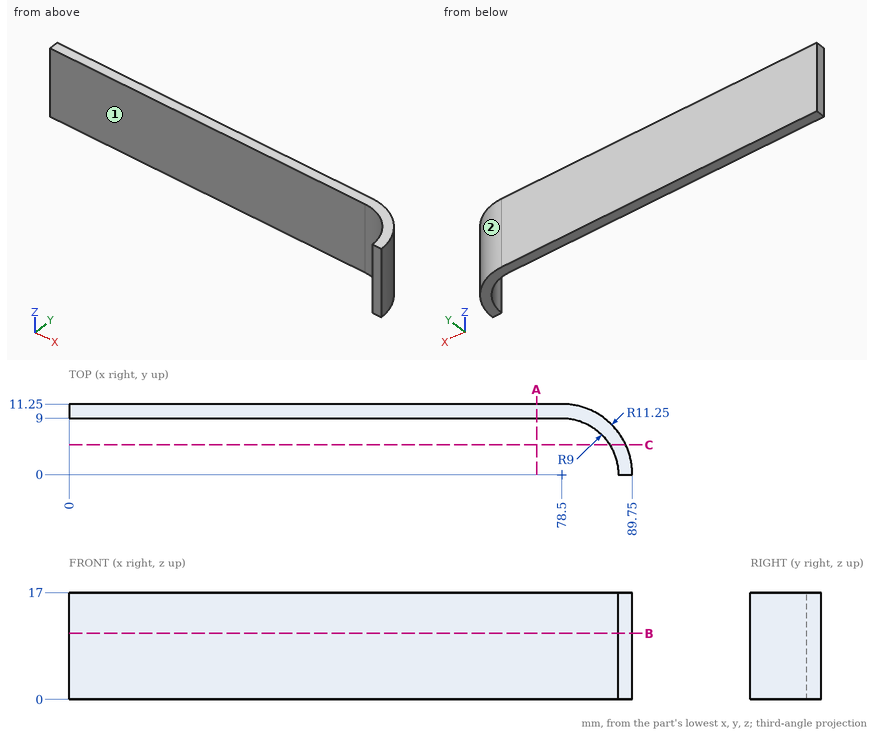
Part print with two shaded views. Sizes in mm from the minimum x, y, z corner. A direction names the side the tool comes from. Round coordinates to 2 decimals unless told otherwise and drop trailing zeros. Order: outer loops, then holes, each group sorted by start corner. A loop starts at its lowest first (then second) coordinate and runs counter-clockwise, first axis right, second up. Notation, with made-up numbers: (78, 36.25) - (126, 36.25) arc R7 cw to (126, 40.25) - close; hole circle Ø4 at (76.25, 8). An arc over 180 degrees is marked (long way). Return JSON: item names as keys, results as strings.
(1) Wall check: probe 1 along Y at (x, z) = (61.5, 1.5); probe 2 along X at (y, z) = (7.25, 11.5); probe 3 along X at (y, z) = (1.75, 8). Give the ranges that are in metal, low to high. Write a range as from..to.
Answer key:
{"probe 1": "y = 9..11.25", "probe 2": "x = 83.83..87.1", "probe 3": "x = 87.33..89.61"}
(2) Tool access for the marked faces 1 and 2: list every direction of +Z, -Z, +X, -X, +Y, -Y with a clear straight run to the whole face (end or side of a thin tool).
Answer key:
{"face 1": "+Z, -Z, -X, -Y", "face 2": "+Z, -Z, +X, +Y"}
(3) Cut at A-A (x = 74.5). Give the cut face in (y, z), then the cut area to 4 significant figures.
Answer key:
{"outline": "(9, 0) - (11.25, 0) - (11.25, 17) - (9, 17) - close", "area": "38.25 mm^2"}
(4) Pin check, flat tips, straight feed: pin 1 Ø5 at (x, z) = (26.5, 11) entering from -Y; pin 2 Ø3 at (y, z) = (1.5, 12) entering from -X. Stop position of each tip, or through.
Answer key:
{"pin 1": "stops at y = 9", "pin 2": "stops at x = 86.99"}
(5) Cut at B-B (z = 10.5). Give the cut face in (x, y).
Answer key:
{"outline": "(0, 9) - (78.5, 9) arc R9 cw to (87.5, 0) - (89.75, 0) arc R11.25 ccw to (78.5, 11.25) - (0, 11.25) - close"}
(6) Cut at C-C (y = 4.75). Give the cut face in (x, z), then the cut area to 3 significant figures.
Answer key:
{"outline": "(86.14, 0) - (88.7, 0) - (88.7, 17) - (86.14, 17) - close", "area": "43.4 mm^2"}
